from build123d import *

# Parameters (mm, degrees)
SKETCH_2_R          = 4
SKETCH_2_R_2        = 2
CUT_EXTRUDE_1_DEPTH = 10


with BuildPart() as part:
    # 草图1 → 旋转1 (revolve)
    with BuildSketch(Plane.XY, mode=Mode.PRIVATE) as revolve_1_sk:
        Polygon((0, 16.5), (-30.5, 16.5), (-30.5, 7.5), (-41, 0), (-37.559069893, 0), (-27.059069893, 7.5), (0, 7.5), align=None)
    revolve(revolve_1_sk.sketch.rotate(Axis((0, 0, 0), (0, 1, 0)), 270), axis=Axis((0, 0, 0), (0, 1, 0)))

    # 草图2 → 切除-拉伸1 (cut)
    with BuildSketch(Plane.XZ.offset(-7.5)):
        with Locations(Location((0, 0, 0), (0, 0, 270))):
            Circle(SKETCH_2_R)
        with Locations(Location((0, 17, 0), (0, 0, 270))):
            Circle(SKETCH_2_R_2)
        with Locations(Location((17, 0, 0), (0, 0, 270))):
            Circle(SKETCH_2_R_2)
        with Locations(Location((0, -17, 0), (0, 0, 270))):
            Circle(SKETCH_2_R_2)
        with Locations(Location((-17, 0, 0), (0, 0, 270))):
            Circle(SKETCH_2_R_2)
    extrude(amount=-CUT_EXTRUDE_1_DEPTH, mode=Mode.SUBTRACT)


solid = part.part
Model file for the job. Use its own axes, mm. A direction names the side the tool comes from. Give positions to 0.01 mm unless a question says otherwise; leave off trailing zeros. Order: outer loops, then holes, each group sorted by start corner. A loop starts at its lowest first (then second) coordinate and runs counter-clockwise, first axis right, second up. Notation, with made-up numbers: M 32.25,-29.5 L 82.25,-29.5 A17 cw 82.25,-9.5 Z; hole C 6.25,31 d7. An arc over 180 degrees is marked long. Put each result on its own line as item: value. Start each with the question number.
(1) Pull direction X, two halves, no side cores. Call faces 1 (the face through (6, 16.5, 0)), 2 (the face through (-27.33, 7.14, 3.59)), 3 (the face through (27.64, 7.03, -14.38)): released by +X, released by -X, zero draft, split by the parting line, or undercut.
(2) Drill centre lines: L1, parallel to X at y = 13.75, z = 0; L2, parallel to Y at x = 17.5, z = 6.5; L3, parallel to X at y = 4.75, z = 18.5. Where is each one in solid material? Low to high. Write a range as [from, to].
(3) Band-saw the part on A-A on z = 0. Give the cut face in (x, y).
(4) Tool access for faces 4 (the face through (-3.905, 11.937, 0.867)), 5 (the face through (0, 7.5, -6)), 6 (the face through (29.775, 11.937, 6.612)): list every direction of +Z, -Z, +X, -X, +Y, -Y with a clear straight run to the whole face (end or side of a thin tool).
(5) Pin check, flat tips, straight feed: pin 1 Ø6.5 at (x, z) = (0, 17) entering from -Y; pin 2 Ø1 at (x, y) = (6, 5) entering from -Z; pin 3 Ø8 at (x, z) = (-21.5, 12.5) entering from -Y; pin 4 Ø3.5 at (x, z) = (17, 0) entering from +Y. Stop position of each tip, or through.
(6) Band-saw the part on B-B on y = 13. Give the cut face in (x, z), then the cut area to 3 significant figures.
(7) Band-saw the part on C-C on y = 5. Give the cut face in (x, z), then the cut area to 3 significant figures.
Results below:
1. face 1: zero draft
1. face 2: undercut
1. face 3: split by the parting line
2. L1: x = [-30.5, -19], [-15, -4], [4, 15], [19, 30.5]
2. L2: y = [7.5, 16.5]
2. L3: x = [-28.94, -24.76], [24.76, 28.94]
3. outline: M -41,0 L -37.56,0 L -27.06,7.5 L -19,7.5 L -19,16.5 L -30.5,16.5 L -30.5,7.5 Z; M -15,7.5 L -4,7.5 L -4,16.5 L -15,16.5 Z; M 4,7.5 L 15,7.5 L 15,16.5 L 4,16.5 Z; M 19,7.5 L 27.06,7.5 L 37.56,0 L 41,0 L 30.5,7.5 L 30.5,16.5 L 19,16.5 Z
4. face 4: +Y, -Y
4. face 5: -Y
4. face 6: +Y
5. pin 1: stops at y = 7.5
5. pin 2: stops at z = -34.18
5. pin 3: stops at y = 6.21
5. pin 4: passes through
6. outline: C 0,0 d61; hole C -17,0 d4; hole C 0,0 d8; hole C 0,-17 d4; hole C 0,17 d4; hole C 17,0 d4
6. area: 2,820 mm2
7. outline: C 0,0 d68; hole C 0,0 d61.12
7. area: 698 mm2
